Input: part model. Units: mm. Frame: model coordinates. Round coordinates to 2 decimals unless told otherwise and drop trailing zeros. Loops run counter-clockwise (first coordinate to the right, second up) from the corner with the lowest first, then second, coordinate; pieces in that order, holes last.
1) First-contact query: pin 1 (1.6 mm diameter, centred on x = 2.5, y = 1.5, fed in from -Z). Flat tip, straight axial feed; report the tip coordinate or a pass-through.
2) Section A-A, the plane z = -24. Return loops of the section in (x, y) (3 decimals).
3) Ray query, line 1 along X through (y, z) = (0.55, -10); line 2 along Z through (x, y) = (3, 1.6); line 3 along X through (y, z) = (2.9, 44). Return the intervals inside material, ascending.
4) Section D-D, the plane x = -22. Return loops of the section in (y, z) (3 decimals).
5) Section C-C, the plane x = 4. Return loops of the section in (y, z) (3 decimals), and give its area (3 significant figures).
6) Section B-B, the plane y = 2.45. Return loops of the section in (x, z), and give its area (3 significant figures).
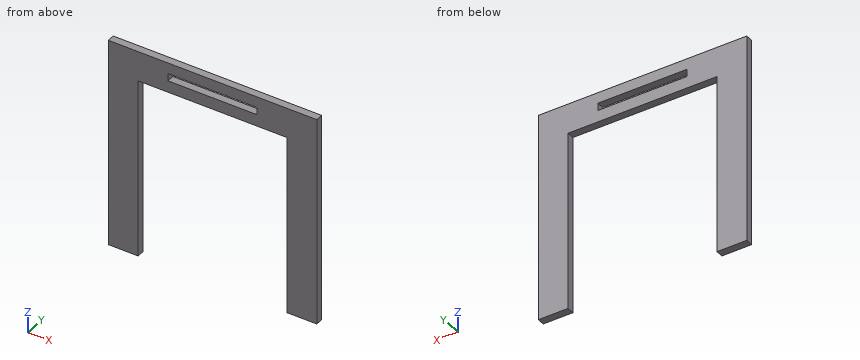
from build123d import *

# Parameters (mm, degrees)
BOSS_EXTRUDE1_DEPTH = 3.175
SKETCH3_W           = 38.1
SKETCH3_H           = 3.175
CUT_EXTRUDE1_DEPTH  = 3.175


with BuildPart() as part:
    # Sketch2 → Boss-Extrude1 (new body)
    with BuildSketch(Plane(origin=(0, 0, 0), x_dir=(1, 0, 0), z_dir=(0, 1, 0))):
        Polygon((-44.199800383, 37.887467748), (-31.499800383, 37.887467748), (-31.499800383, -38.312532252), (32.000199617, -38.312532252), (32.000199617, 37.887467748), (44.700199617, 37.887467748), (44.700199617, -38.312532252), (44.700199617, -51.012532252), (-44.199800383, -51.012532252), (-44.199800383, -38.312532252), align=None)
    extrude(amount=BOSS_EXTRUDE1_DEPTH)

    # Sketch3 → Cut-Extrude1 (cut)
    with BuildSketch(Plane(origin=(0, 3.175, 0), x_dir=(1, 0, 0), z_dir=(0, 1, 0))):
        with Locations((0.250199617, -44.853032252)):
            Rectangle(SKETCH3_W, SKETCH3_H)
    extrude(amount=-CUT_EXTRUDE1_DEPTH, mode=Mode.SUBTRACT)


solid = part.part
Final values:
1. pin 1: stops at z = 38.31
2. outline: (-44.2, 0) - (-31.5, 0) - (-31.5, 3.175) - (-44.2, 3.175) - close; (32, 0) - (44.7, 0) - (44.7, 3.175) - (32, 3.175) - close
3. line 1: x = -44.2 to -31.5, 32 to 44.7
3. line 2: z = 38.31 to 43.27, 46.44 to 51.01
3. line 3: x = -44.2 to -18.8, 19.3 to 44.7
4. outline: (0, 38.313) - (3.175, 38.313) - (3.175, 51.013) - (0, 51.013) - close
5. outline: (0, 38.313) - (3.175, 38.313) - (3.175, 43.266) - (0, 43.266) - close; (0, 46.441) - (3.175, 46.441) - (3.175, 51.013) - (0, 51.013) - close
5. area: 30.2 mm2
6. outline: (-44.2, -37.89) - (-31.5, -37.89) - (-31.5, 38.31) - (32, 38.31) - (32, -37.89) - (44.7, -37.89) - (44.7, 51.01) - (-44.2, 51.01) - close; hole (-18.8, 43.27) - (19.3, 43.27) - (19.3, 46.44) - (-18.8, 46.44) - close
6. area: 2,940 mm2
